For this review, use the dimensioned drawing (mm, ordinates from the lowest corner) and the shaded views. A direction names the side the tool comes from. Round coordinates to 2 decimals unless told otherwise and drop trailing zeros. Loops run counter-clockwise (first coordinate to the right, second up) from the corner with the lowest first, then second, coordinate; pieces in that order, holes last. Notation, with made-up numbers: (-10, 33.25) - (13, 33.25) arc R27 cw to (13, 55.25) - close; hole circle Ø6 at (77, -29.5). An arc over 180 degrees is marked (long way). Answer as CSV lines item,"result". Start each with the question number.
(1) Consider section D-D (z = 55.5). Give the boundary of the cut face in (x, y).
(2) Consider section B-B (y = 22). Give the boundary of the cut face in (x, z).
(3) For P1, Ø6, axis at y = 3.5, z = 30, coming from the +X side; P2, Ø1, axis at y = 16.5, z = 9, coming from the -X side; P3, Ø3, axis at x = 40.5, z = 61.5, coming from the +Y side; P4, Ø4.5, axis at y = 26, z = 25, coming from the +X side, all flat-tipped, find the tip position at first contact; note any pin that passes through.
(4) Wall thickness on L1, parallel to X at y = 1.5, z = 7; L2, parallel to Y at x = 7, z = 35; L3, parallel to X at y = 5.5, z = 33.5: over which ranges is each line inside the solid? List them lowest first.
(5) Mouldability with a two-part tool opening along X and no side actions: class the marked faces 1, 2 and 3 as released by +X, released by -X, zero draft, split by the parting line, or undercut.
(6) Consider section C-C (x = 7.5). Give the boundary of the cut face in (y, z).
(7) Consider section A-A (z = 19). Give the boundary of the cut face in (x, y).
(8) For the marked faces 4, 5 and 6, list the 3-axis set-ups (+Z, -Z, +X, -X, +Y, -Y) from which the entire face can be reached by the end or side of a thin tool; tool diameter is ignored.
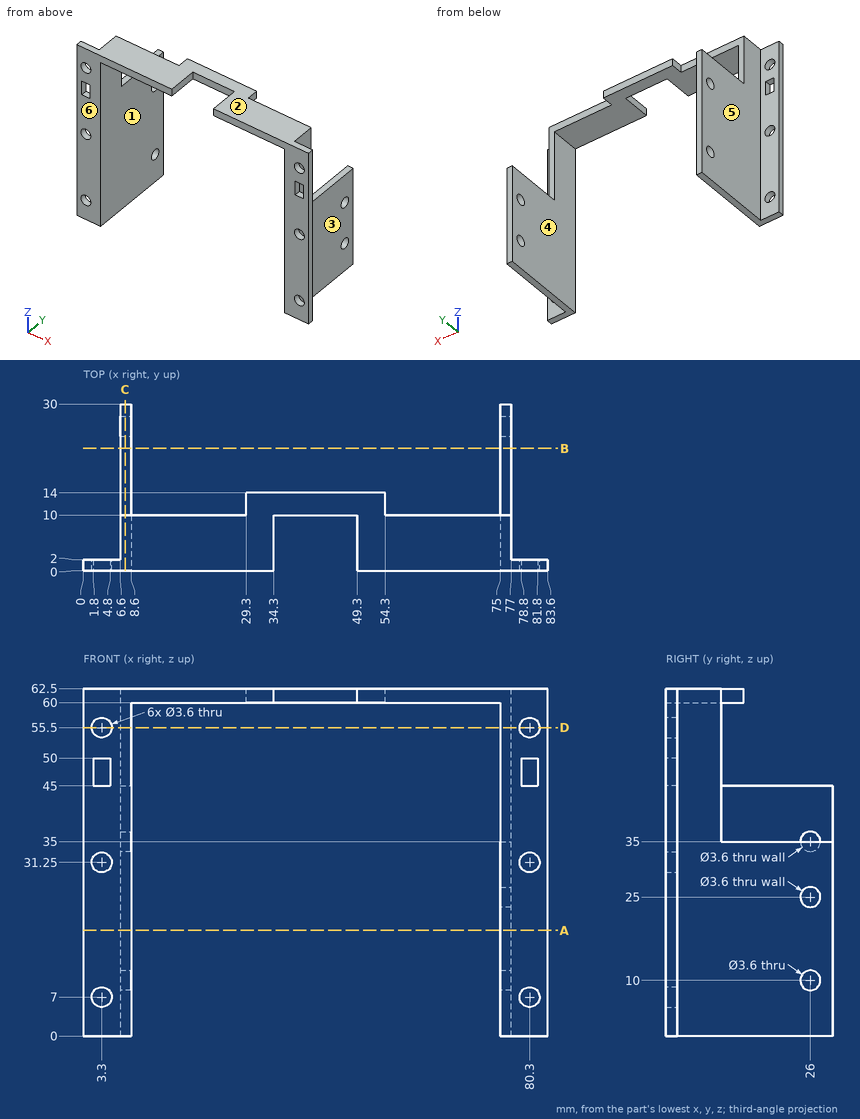
Determined:
1,outline,"(0, 0) - (1.5, 0) - (1.5, 2) - (0, 2) - close; (5.1, 0) - (8.6, 0) - (8.6, 10) - (6.6, 10) - (6.6, 2) - (5.1, 2) - close; (75, 0) - (78.5, 0) - (78.5, 2) - (77, 2) - (77, 10) - (75, 10) - close; (82.1, 0) - (83.6, 0) - (83.6, 2) - (82.1, 2) - close"
2,outline,"(6.6, 0) - (8.6, 0) - (8.6, 45) - (6.6, 45) - close; (75, 0) - (77, 0) - (77, 35) - (75, 35) - close"
3,P1,"stops at x = 83.6"
3,P2,"stops at x = 6.6"
3,P3,"stops at y = 14"
3,P4,"stops at x = 77"
4,L1,"x = 0 to 1.5, 5.1 to 8.6, 75 to 78.5, 82.1 to 83.6"
4,L2,"y = 0 to 24.2, 27.8 to 30"
4,L3,"x = 6.6 to 8.6, 75 to 77"
5,face 1,"undercut"
5,face 2,"zero draft"
5,face 3,"released by +X"
6,outline,"(0, 0) - (30, 0) - (30, 45) - (10, 45) - (10, 62.5) - (0, 62.5) - close; hole circle Ø3.6 at (26, 10); hole circle Ø3.6 at (26, 35)"
7,outline,"(0, 0) - (8.6, 0) - (8.6, 30) - (6.6, 30) - (6.6, 2) - (0, 2) - close; (75, 0) - (83.6, 0) - (83.6, 2) - (77, 2) - (77, 30) - (75, 30) - close"
8,face 4,"-Z, +Y, -Y"
8,face 5,"+Z, -Z, -X, +Y"
8,face 6,"+Z, -Z, +X, -X, -Y"
